Could you check a few things on this model? Use its own coordinates, in mm. Give positions to 0.01 mm unless a question says otherwise; leave off trailing zeros. Order: outer loops, then holes, each group sorted by start corner. A loop starts at its lowest first (then second) coordinate and runs counter-clockwise, first axis right, second up. Notation, with made-up numbers: (82.5, 52.25) -> (126.5, 52.25) arc R31 ccw to (126.5, 81.25) -> close; hole circle Ø8 at (13, 43). An arc over 180 degrees is marked (long way). Use one line per item in the form item = value. Start each with the question number.
from build123d import *

# Parameters (mm, degrees)
EXTRUDE_1_DEPTH     = 8
FILLET_1_R          = 3
FILLET_2_R          = 5
SKETCH_2_R          = 1.75
SKETCH_2_R_2        = 5.525
CUT_EXTRUDE_1_DEPTH = 10
SKETCH_3_R          = 9.5
CUT_EXTRUDE_2_DEPTH = 497.999889336


with BuildPart() as part:
    # 草图1 → 凸台-拉伸1 (new body)
    with BuildSketch(Plane.XY):
        Polygon((0, 0), (50, 0), (116.65, -5), (376.65, -5), (443.3, 0), (493.3, 0), (493.3, -60), (443.3, -60), (376.65, -55), (116.65, -55), (50, -60), (0, -60), align=None)
        Polygon((116.65, -30), (146.65, -20), (176.65, -30), (146.65, -40), align=None, mode=Mode.SUBTRACT)
        Polygon((216.65, -30), (246.65, -20), (276.65, -30), (246.65, -40), align=None, mode=Mode.SUBTRACT)
        Polygon((316.65, -30), (346.65, -20), (376.65, -30), (346.65, -40), align=None, mode=Mode.SUBTRACT)
    extrude(amount=EXTRUDE_1_DEPTH)

    # 圆角1
    fillet_1_edges = [part.edges().sort_by_distance(p)[0] for p in [
        (216.65, -30, 4),
        (246.65, -40, 4),
        (276.65, -30, 4),
        (246.65, -20, 4),
        (116.65, -30, 4),
        (146.65, -40, 4),
        (176.65, -30, 4),
        (146.65, -20, 4),
        (316.65, -30, 4),
        (346.65, -40, 4),
        (376.65, -30, 4),
        (346.65, -20, 4),
    ]]
    fillet(fillet_1_edges, radius=FILLET_1_R)

    # 圆角2
    fillet_2_edges = [part.edges().sort_by_distance(p)[0] for p in [
        (0, 0, 4),
        (493.3, 0, 4),
        (493.3, -60, 4),
        (0, -60, 4),
    ]]
    fillet(fillet_2_edges, radius=FILLET_2_R)

    # 草图2 → 切除-拉伸1 (cut)
    with BuildSketch(Plane.XY.offset(8)):
        with Locations((4.75, -4)):
            Circle(SKETCH_2_R)
        with Locations((18.75, -4)):
            Circle(SKETCH_2_R)
        with Locations((18.75, -56)):
            Circle(SKETCH_2_R)
        with Locations((4.75, -56)):
            Circle(SKETCH_2_R)
        with Locations((21.3, -30)):
            Circle(SKETCH_2_R_2)
        with Locations((488.55, -4)):
            Circle(SKETCH_2_R)
        with Locations((474.55, -4)):
            Circle(SKETCH_2_R)
        with Locations((474.55, -56)):
            Circle(SKETCH_2_R)
        with Locations((488.55, -56)):
            Circle(SKETCH_2_R)
        with Locations((472, -30)):
            Circle(SKETCH_2_R_2)
    extrude(amount=-CUT_EXTRUDE_1_DEPTH, mode=Mode.SUBTRACT)

    # 草图3 → 切除-拉伸2 (cut, through all)
    with BuildSketch(Plane.XY.offset(8)):
        with Locations((60, -30)):
            Circle(SKETCH_3_R)
    extrude(amount=-CUT_EXTRUDE_2_DEPTH, mode=Mode.SUBTRACT)


solid = part.part
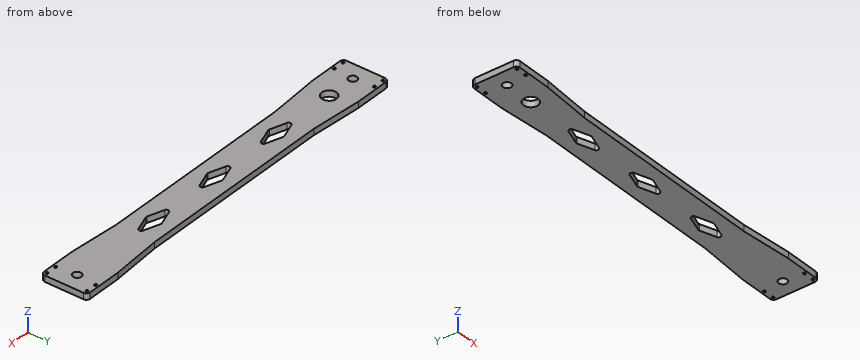
(1) Please list where these lines run through material, in increasing order: probe 1 along Y at (x, z) = (4.75, 4); probe 2 along Y at (x, z) = (18.75, 6.25); probe 3 along Y at (x, z) = (472, 4.25) (3 decimals).
(2) Imagine slicing it at C-C (z = 4.25). Give the number of separate pieces and of enclosed holes in the cut face, plus the area to 3 significant figures.
(3) Imagine slicing it at A-A (x = 60). Write out the boundary of the cut face in (y, z).
(4) I'm going to push flat-ended pins straight in: pin 1 Ø2 at (x, y) = (488.55, -56) entering from +Z; pin 2 Ø2.5 at (x, z) = (244.5, 5) entering from -Y; pin 3 Ø1.5 at (x, z) = (327, 5.5) entering from +Y; pin 4 Ø1 at (x, z) = (407.5, 5.5) entering from -Y. Where does each tip first touch, or does it pass through?
(5) Imagine slicing it at B-B (x = 319). Write out the boundary of the cut face in (y, z), plus the area to 3 significant figures.
Calculated:
q1.probe_1 = -59.99 to -57.75, -54.25 to -5.75, -2.25 to -0.01
q1.probe_2 = -60 to -57.75, -54.25 to -34.9, -25.1 to -5.75, -2.25 to 0
q1.probe_3 = -60 to -35.525, -24.475 to 0
q2.separate_pieces = 1
q2.enclosed_holes = 14
q2.area = 24,100 mm2
q3.outline = (-59.25, 0) -> (-39.5, 0) -> (-39.5, 8) -> (-59.25, 8) -> close; (-20.5, 0) -> (-0.75, 0) -> (-0.75, 8) -> (-20.5, 8) -> close
q4.pin_1 = through
q4.pin_2 = -55
q4.pin_3 = -5
q4.pin_4 = -57.35
q5.outline = (-55, 0) -> (-5, 0) -> (-5, 8) -> (-55, 8) -> close
q5.area = 400 mm2
